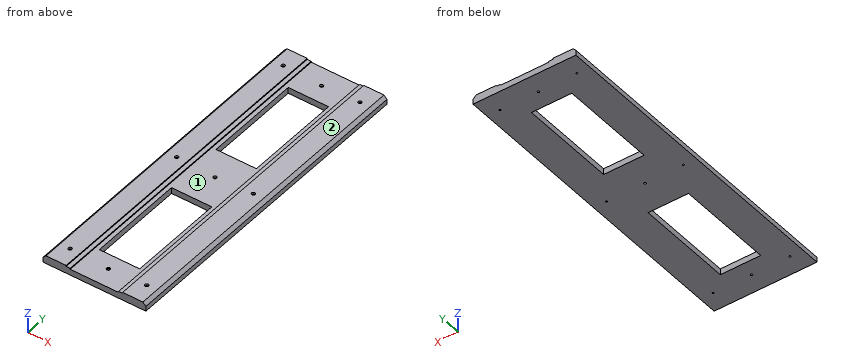
```python
from build123d import *

# Parameters (mm, degrees)
F0_W                   = 323.799
F0_H                   = 1018.061
F0_W_2                 = 127
F0_H_2                 = 304.8
F1_DEPTH               = 25.4
F2_W                   = 177.8
F2_H                   = 1077.8446237831
F3_DEPTH               = 3.175
F4_W                   = 152.4
F4_H                   = 1094.5154423737
F5_DEPTH               = 3.175
F6_SIZE                = 9.525
F8_D                   = 6.6
F8_DEPTH               = 25
F8_CBORE_D             = 11.25
F8_CBORE_DEPTH         = 6
F8_TIP                 = 1.9828400428
F10_D                  = 6.6
F10_DEPTH              = 25
F10_CBORE_D            = 11.25
F10_CBORE_DEPTH        = 6
F10_TIP                = 1.9828400428
F13_D                  = 6.6
F13_CBORE_D            = 11.25
F13_CBORE_DEPTH        = 6
F13_ON_F12_D           = 6.6
F13_ON_F12_CBORE_D     = 11.25
F13_ON_F12_CBORE_DEPTH = 6


# Not quite as in the source:
# - a feature names something its author has since deleted; it is built from what else it names


with BuildPart() as f1:
    # F0 (on Top) → F1 (new body)
    with BuildSketch(Plane.XY):
        with Locations((-161.8995, 509.0305)):
            Rectangle(F0_W, F0_H)
        with Locations((-162.103, 258.488)):
            Rectangle(F0_W_2, F0_H_2, mode=Mode.SUBTRACT)
        with Locations((-162.103, 751.124)):
            Rectangle(F0_W_2, F0_H_2, mode=Mode.SUBTRACT)
    extrude(amount=F1_DEPTH)

    # F2 (on face) → F3 (cut)
    with BuildSketch(Plane.XY.offset(25.4)):
        with Locations((-162.103, 495.1518476009)):
            Rectangle(F2_W, F2_H)
    extrude(amount=-F3_DEPTH, mode=Mode.SUBTRACT)

    # F4 (on face) → F5 (cut)
    with BuildSketch(Plane.XY.offset(22.225)):
        with Locations((-162.103, 504.4111407595)):
            Rectangle(F4_W, F4_H)
    extrude(amount=-F5_DEPTH, mode=Mode.SUBTRACT)

    # F6
    f6_edges = [f1.edges().sort_by_distance(p)[0] for p in [
        (-323.799, 509.0305, 25.4),
        (0, 509.0305, 25.4),
    ]]
    chamfer(f6_edges, length=F6_SIZE)

    # F8
    with Locations(Plane.XY.offset(25.4)):
        with Locations((-41.16, 59.0305), (-41.16, 509.0305), (-41.16, 959.0305)):
            CounterBoreHole(F8_D / 2, F8_CBORE_D / 2, F8_CBORE_DEPTH, depth=F8_DEPTH)
            with Locations((0, 0, -(F8_DEPTH + F8_TIP / 2))):  # 118° drill point
                Cone(0, F8_D / 2, F8_TIP, mode=Mode.SUBTRACT)

    # F10
    with Locations(Plane.XY.offset(25.4)):
        with Locations((-282.6385, 59.0305), (-282.6385, 509.0305), (-282.6385, 959.0305)):
            CounterBoreHole(F10_D / 2, F10_CBORE_D / 2, F10_CBORE_DEPTH, depth=F10_DEPTH)
            with Locations((0, 0, -(F10_DEPTH + F10_TIP / 2))):  # 118° drill point
                Cone(0, F10_D / 2, F10_TIP, mode=Mode.SUBTRACT)

    # F13 (through all)
    with Locations(Plane.XY.offset(22.225)):
        with Locations((-161.89925, 59.0305)):
            CounterBoreHole(F13_D / 2, F13_CBORE_D / 2, F13_CBORE_DEPTH)

    # F13 on F12 (through all)
    with Locations(Plane.XY.offset(19.05)):
        with Locations((-161.89925, 509.0305), (-161.89925, 959.0305)):
            CounterBoreHole(F13_ON_F12_D / 2, F13_ON_F12_CBORE_D / 2, F13_ON_F12_CBORE_DEPTH)


solid = f1.part
```
Can you work these out from the model? Positions are in its coordinate system, mm. Face numbers are marked on the shaded views. Give positions to 0.01 mm unless a question says otherwise; leave off trailing zeros. Order: outer loops, then holes, each group sorted by start corner. A loop starts at its lowest first (then second) coordinate and runs counter-clockwise, first axis right, second up. Notation, with made-up numbers: (15.5, 23.25) - (65.5, 23.25) arc R8 cw to (65.5, 28.25) - close; hole circle Ø3 at (23, 7). An arc over 180 degrees is marked (long way). Use a Markdown table: item, result. Add a question column.
Q1. I'm going to push flat-ended pins straight in: pin 1 (3.5 mm diameter, centred on x = -162.5, y = 510, fed in from +Z); pin 2 (4 mm diameter, centred on y = 782, z = 22.5, fed in from +X) (3 decimals); pin 3 (3.5 mm diameter, centred on y = 541, z = 20.5, fed in from -X); pin 4 (9 mm diameter, centred on x = -161.9, y = 509.03, fed in from +Z). Where does each tip first touch, or does it pass through?
Q2. If we section it at A-A on y = 362.5: Write out the boundary of the cut face in (x, z) (3 decimals), plus the area to 3 significant figures.
Q3. If we mould it in two halves opening along X, with no side actions, what happens to the marked faces 1 and 2? For each: released by +X, released by -X, zero draft, split by the parting line, or undercut.
Q4. Please list where these lines run through material, in increasing order: line 1 along Y through (x, z) = (-181.5, 13.25); line 2 along Y through (x, z) = (-41.16, 10.25); line 3 along X through (y, z) = (654, 5.5).
Q5. If we section it at B-B on x = -199: Write out the boundary of the cut face in (y, z), plus the area to 3 significant figures.
Q6. If we section it at C-C on z = 8: Count the separate pieces of the cut face and the enclosed holes in it, plus the area to 3 significant figures.
Answers follow:
| question | item | result |
|---|---|---|
| 1 | pin 1 | passes through |
| 1 | pin 2 | stops at x = -4.625 |
| 1 | pin 3 | stops at x = -320.92 |
| 1 | pin 4 | stops at z = 13.05 |
| 2 | outline | (-323.799, 0) - (-225.603, 0) - (-225.603, 19.05) - (-238.303, 19.05) - (-238.303, 22.225) - (-251.003, 22.225) - (-251.003, 25.4) - (-314.274, 25.4) - (-323.799, 15.875) - close; (-98.603, 0) - (0, 0) - (0, 15.875) - (-9.525, 25.4) - (-73.203, 25.4) - (-73.203, 22.225) - (-85.903, 22.225) - (-85.903, 19.05) - (-98.603, 19.05) - close |
| 2 | area | 4,670 mm^2 |
| 3 | face 1 | undercut |
| 3 | face 2 | zero draft |
| 4 | line 1 | y = 0 to 106.09, 410.89 to 598.72, 903.52 to 1018.06 |
| 4 | line 2 | y = 0 to 55.73, 62.33 to 505.73, 512.33 to 955.73, 962.33 to 1018.06 |
| 4 | line 3 | x = -323.8 to -225.6, -98.6 to 0 |
| 5 | outline | (0, 0) - (106.09, 0) - (106.09, 19.05) - (0, 19.05) - close; (410.89, 0) - (598.72, 0) - (598.72, 19.05) - (410.89, 19.05) - close; (903.52, 0) - (1018.06, 0) - (1018.06, 19.05) - (903.52, 19.05) - close |
| 5 | area | 7,780 mm^2 |
| 6 | separate pieces | 1 |
| 6 | enclosed holes | 11 |
| 6 | area | 252,000 mm^2 |
